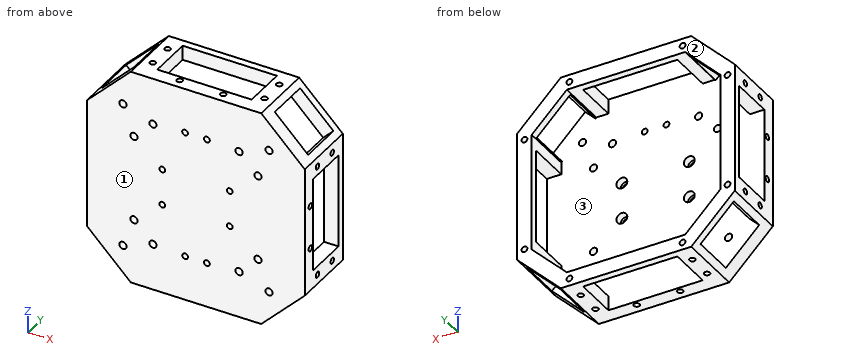
from build123d import *

# Parameters (mm, degrees)
BOSS_EXTRUDE1_DEPTH                     = 90
CUT_EXTRUDE2_DEPTH                      = 70
SKETCH6_W                               = 130
SKETCH6_H                               = 60
CUT_EXTRUDE3_DEPTH                      = 70
CIRPATTERN1_COUNT                       = 4
SKETCH7_W                               = 65
SKETCH7_H                               = 60
CUT_EXTRUDE4_DEPTH                      = 382.764068712
CIRPATTERN2_COUNT                       = 4
F_1_0MM_DOWEL_HOLE1_D                   = 10
F_1_0MM_DOWEL_HOLE2_D                   = 8
MIRROR2_COPY_1_D                        = 10
MIRROR2_COPY_2_D                        = 8
CBORE_FOR_M5_HEX_HEAD_BOLT1_D           = 8
CBORE_FOR_M5_HEX_HEAD_BOLT1_CBORE_D     = 15
CBORE_FOR_M5_HEX_HEAD_BOLT1_CBORE_DEPTH = 10
F_1_0MM_DOWEL_HOLE5_D                   = 8
F_1_0MM_DOWEL_HOLE5_DEPTH               = 20
F_1_0MM_DOWEL_HOLE10_D                  = 8
F_1_0MM_DOWEL_HOLE10_DEPTH              = 10
F_1_0MM_DOWEL_HOLE11_D                  = 8
F_1_0MM_DOWEL_HOLE11_DEPTH              = 10


with BuildPart() as part:
    # Sketch1 → Boss-Extrude1 (new body)
    with BuildSketch(Plane(origin=(0, 0, 0), x_dir=(1, 0, 0), z_dir=(0, 1, 0))):
        Polygon((-150, 89.895923599), (-89.895923599, 150), (89.895923599, 150), (150, 89.895923599), (150, -89.895923599), (89.895923599, -150), (-89.895923599, -150), (-150, -89.895923599), align=None)
    extrude(amount=BOSS_EXTRUDE1_DEPTH)

    # Sketch2 → Cut-Extrude2 (cut)
    with BuildSketch(Plane(origin=(0, 90, 0), x_dir=(1, 0, 0), z_dir=(0, 1, 0))):
        Polygon((-130, -81.611652352), (-130, 81.611652352), (-81.611652352, 130), (81.611652352, 130), (130, 81.611652352), (130, -81.611652352), (81.611652352, -130), (-81.611652352, -130), align=None)
    extrude(amount=-CUT_EXTRUDE2_DEPTH, mode=Mode.SUBTRACT)

    # Sketch6 → Cut-Extrude3 (cut)
    with BuildSketch(Plane(origin=(150, 0, 0), x_dir=(0, 0, -1), z_dir=(1, 0, 0))):
        with Locations((0, 50)):
            Rectangle(SKETCH6_W, SKETCH6_H)
    cut_extrude3 = extrude(amount=-CUT_EXTRUDE3_DEPTH, mode=Mode.SUBTRACT)

    # CirPattern1: Cut-Extrude3 ×4 about axis
    cirpattern1_axis = Axis((0, 0, 0), (0, 1, 0))
    for i in range(1, CIRPATTERN1_COUNT):
        add(cut_extrude3.rotate(cirpattern1_axis, i * 360 / CIRPATTERN1_COUNT), mode=Mode.SUBTRACT)

    # Sketch7 → Cut-Extrude4 (cut, through all)
    with BuildSketch(Plane(origin=(119.9479618, 0, 119.9479618), x_dir=(0.707106781, 0, -0.707106781), z_dir=(0.707106781, 0, 0.707106781))):
        with Locations((0, 50)):
            Rectangle(SKETCH7_W, SKETCH7_H)
    cut_extrude4 = extrude(amount=-CUT_EXTRUDE4_DEPTH, mode=Mode.SUBTRACT)

    # CirPattern2: Cut-Extrude4 ×4 about axis
    cirpattern2_axis = Axis((0, 20, 0), (0, -1, 0))
    for i in range(1, CIRPATTERN2_COUNT):
        add(cut_extrude4.rotate(cirpattern2_axis, i * 360 / CIRPATTERN2_COUNT), mode=Mode.SUBTRACT)

    # Ø1.0mm Dowel Hole1 (through all)
    with Locations(Plane(origin=(0, 20, 0), x_dir=(1, 0, 0), z_dir=(0, 1, 0))):
        with Locations((-100.72, -100.72), (-85.48, -59.39), (-59.39, -85.48)):
            f_1_0mm_dowel_hole1 = Hole(F_1_0MM_DOWEL_HOLE1_D / 2)

    # Ø1.0mm Dowel Hole2 (through all)
    with Locations(Plane(origin=(0, 20, 0), x_dir=(1, 0, 0), z_dir=(0, 1, 0))):
        with Locations((-15.01, -88)):
            f_1_0mm_dowel_hole2 = Hole(F_1_0MM_DOWEL_HOLE2_D / 2)

    # Mirror1: Ø1.0mm Dowel Hole1, Ø1.0mm Dowel Hole2 across plane
    add(f_1_0mm_dowel_hole1.mirror(Plane.XY), mode=Mode.SUBTRACT)
    add(f_1_0mm_dowel_hole2.mirror(Plane.XY), mode=Mode.SUBTRACT)

    # Mirror2: Ø1.0mm Dowel Hole1, Ø1.0mm Dowel Hole2 across plane
    add(f_1_0mm_dowel_hole1.mirror(Plane(origin=(0, 0, 0), x_dir=(0, 0, 1), z_dir=(1, 0, 0))), mode=Mode.SUBTRACT)
    add(f_1_0mm_dowel_hole2.mirror(Plane(origin=(0, 0, 0), x_dir=(0, 0, 1), z_dir=(1, 0, 0))), mode=Mode.SUBTRACT)

    # Mirror2 copy 1 (through all)
    with Locations(Plane(origin=(0, 20, 0), x_dir=(-1, 0, 0), z_dir=(0, 1, 0))):
        with Locations((-100.72, -100.72), (-85.48, -59.39), (-59.39, -85.48)):
            Hole(MIRROR2_COPY_1_D / 2)

    # Mirror2 copy 2 (through all)
    with Locations(Plane(origin=(0, 20, 0), x_dir=(-1, 0, 0), z_dir=(0, 1, 0))):
        with Locations((-15.01, -88)):
            Hole(MIRROR2_COPY_2_D / 2)

    # CBORE for M5 Hex Head Bolt1 (through all)
    with Locations(Plane(origin=(0, 20, 0), x_dir=(1, 0, 0), z_dir=(0, 1, 0))):
        with Locations((-46.51, -25.01), (46.49, -25.01)):
            cbore_for_m5_hex_head_bolt1 = CounterBoreHole(CBORE_FOR_M5_HEX_HEAD_BOLT1_D / 2, CBORE_FOR_M5_HEX_HEAD_BOLT1_CBORE_D / 2, CBORE_FOR_M5_HEX_HEAD_BOLT1_CBORE_DEPTH)

    # Mirror3: CBORE for M5 Hex Head Bolt1 across plane
    add(cbore_for_m5_hex_head_bolt1.mirror(Plane.XY), mode=Mode.SUBTRACT)

    # Ø1.0mm Dowel Hole5
    with Locations(Plane(origin=(0, 90, 0), x_dir=(1, 0, 0), z_dir=(0, 1, 0))):
        with Locations((-140.01, -78.01), (-78.01, -140.01), (77.99, -140.01), (139.99, -78.01)):
            f_1_0mm_dowel_hole5 = Hole(F_1_0MM_DOWEL_HOLE5_D / 2, depth=F_1_0MM_DOWEL_HOLE5_DEPTH)

    # Mirror4: Ø1.0mm Dowel Hole5 across plane
    add(f_1_0mm_dowel_hole5.mirror(Plane.XY), mode=Mode.SUBTRACT)

    # Ø1.0mm Dowel Hole10
    with Locations(Plane(origin=(150, 0, 0), x_dir=(0, 0, -1), z_dir=(1, 0, 0))):
        with Locations((-77, 65), (-77, 30), (-30, 13), (30, 13), (77, 30), (77, 65)):
            f_1_0mm_dowel_hole10 = Hole(F_1_0MM_DOWEL_HOLE10_D / 2, depth=F_1_0MM_DOWEL_HOLE10_DEPTH)

    # Mirror5: Ø1.0mm Dowel Hole10 across plane
    add(f_1_0mm_dowel_hole10.mirror(Plane(origin=(0, 0, 0), x_dir=(0, 0, 1), z_dir=(1, 0, 0))), mode=Mode.SUBTRACT)

    # Ø1.0mm Dowel Hole11
    with Locations(Plane.XY.offset(150)):
        with Locations((-77, 65), (-77, 30), (-30, 13), (30, 13), (77, 30), (77, 65)):
            f_1_0mm_dowel_hole11 = Hole(F_1_0MM_DOWEL_HOLE11_D / 2, depth=F_1_0MM_DOWEL_HOLE11_DEPTH)

    # Mirror6: Ø1.0mm Dowel Hole11 across plane
    add(f_1_0mm_dowel_hole11.mirror(Plane.XY), mode=Mode.SUBTRACT)


solid = part.part
Source: CAD feature listing. Evaluate the final solid. Frame: model axes, mm. Face numbers are marked on the shaded views. Coordinates: 2 decimals unless noted, no trailing zeros. Order: outer loops, then holes, each group sorted by start corner. A loop starts at its lowest first (then second) coordinate and runs counter-clockwise, first axis right, second up.
Item 1: Cut plane A-A (x = -30). Return loops of the section in (y, z).
Output values:
outline: (0, -150) - (9, -150) - (9, -140) - (17, -140) - (17, -150) - (20, -150) - (20, 150) - (17, 150) - (17, 140) - (9, 140) - (9, 150) - (0, 150) - close; (80, -150) - (90, -150) - (90, -130) - (80, -130) - close; (80, 130) - (90, 130) - (90, 150) - (80, 150) - close
Item 2: Cut plane C-C (z = -59.39). Return loops of the section in (x, y).
Output values:
outline: (-150, 0) - (-90.48, 0) - (-90.48, 20) - (-150, 20) - close; (-150, 80) - (-130, 80) - (-130, 90) - (-150, 90) - close; (-80.48, 0) - (80.48, 0) - (80.48, 20) - (-80.48, 20) - close; (90.48, 0) - (150, 0) - (150, 20) - (90.48, 20) - close; (130, 80) - (150, 80) - (150, 90) - (130, 90) - close
Item 3: Cut plane B-B (z = -13.5). Return loops of the section in (x, y).
Output values:
outline: (-150, 0) - (150, 0) - (150, 20) - (-150, 20) - close; (-150, 80) - (-130, 80) - (-130, 90) - (-150, 90) - close; (130, 80) - (150, 80) - (150, 90) - (130, 90) - close
Item 4: Cut plane D-D (y = 84.5). Count the separate pieces of the cut face and the enclosed holes in it, plus the area to 3 significant figures.
Output values:
separate pieces: 1
enclosed holes: 9
area: 19,500 mm2
Item 5: Pull-direction query (Y, two-part tool) for the marked faces 1, 2 and 3; classes: pulls with the +Y half, pulls with the -Y half, needs draft (parallel to the pull), parting line crosses it, or undercut.
Output values:
face 1: pulls with the -Y half
face 2: pulls with the +Y half
face 3: undercut
Item 6: Material intervals for line 1 (Z direction, x = -78.5, y = 80.5); line 2 (Y direction, x = 148, z = -30); line 3 (X direction, y = 8, z = -59), sorted ascending.
Output values:
line 1: z = -150 to -143.98, -136.04 to -130, 130 to 136.04, 143.98 to 150
line 2: y = 0 to 9, 17 to 20, 80 to 90
line 3: x = -150 to -90.46, -80.5 to 80.5, 90.46 to 150
Item 7: First-contact query: P1, Ø6.5, axis at y = 63.5, z = 77, coming from the +X side; P2, Ø3, axis at x = -92, z = -9, coming from the +Y side; P3, Ø5, axis at x = -77, y = 30, coming from the +Z side; P4, Ø5, axis at y = 65, z = -77, coming from the +X side. Flat tips, straight axial feed; report the tip coordinate or a pass-through.
Output values:
P1: stops at x = 150
P2: stops at y = 20
P3: stops at z = 140
P4: stops at x = 140
